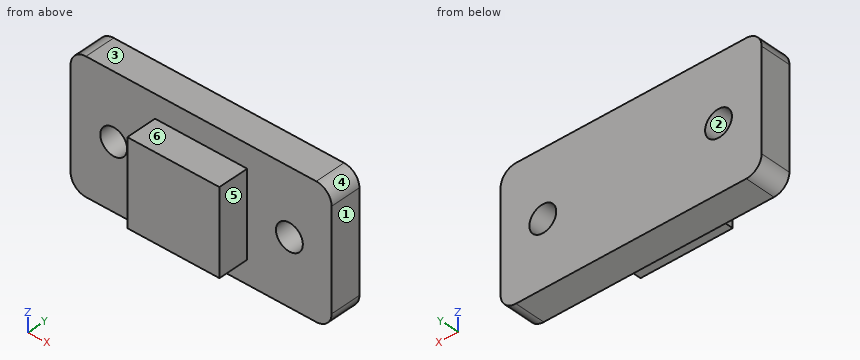
```python
from build123d import *

# Parameters (mm, degrees)
SKETCH1_W           = 12
SKETCH1_H           = 11
BOSS_EXTRUDE1_DEPTH = 4
SKETCH2_W           = 34
SKETCH2_H           = 17
BOSS_EXTRUDE2_DEPTH = 4
SKETCH3_R           = 1.75
CUT_EXTRUDE1_DEPTH  = 5
FILLET1_R           = 2


with BuildPart() as part:
    # Sketch1 → Boss-Extrude1 (new body)
    with BuildSketch(Plane(origin=(0, 0, 0), x_dir=(1, 0, 0), z_dir=(0, 1, 0))):
        with Locations((6, -5.5)):
            Rectangle(SKETCH1_W, SKETCH1_H)
    extrude(amount=BOSS_EXTRUDE1_DEPTH)

    # Sketch2 → Boss-Extrude2 (add)
    with BuildSketch(Plane(origin=(0, 4, 0), x_dir=(1, 0, 0), z_dir=(0, 1, 0))):
        with Locations((6, -5.5)):
            Rectangle(SKETCH2_W, SKETCH2_H)
    extrude(amount=BOSS_EXTRUDE2_DEPTH)

    # Sketch3 → Cut-Extrude1 (cut, through all)
    with BuildSketch(Plane.XZ.offset(-4)):
        with Locations((-5.385399537, 5.5)):
            Circle(SKETCH3_R)
        with Locations((17.5, 5.5)):
            Circle(SKETCH3_R)
    extrude(amount=-CUT_EXTRUDE1_DEPTH, mode=Mode.SUBTRACT)

    # Fillet1
    fillet1_edges = [part.edges().sort_by_distance(p)[0] for p in [
        (23, 6, 14),
        (23, 6, -3),
        (-11, 6, -3),
        (-11, 6, 14),
    ]]
    fillet(fillet1_edges, radius=FILLET1_R)


solid = part.part
```
For this review, take the finished solid that the model builds, in its own axes (mm). Face numbers are marked on the shaded views. A direction names the side the tool comes from. Give positions to 0.01 mm unless a question says otherwise; leave off trailing zeros. Loops run counter-clockwise (first coordinate to the right, second up) from the corner with the lowest first, then second, coordinate; pieces in that order, holes last. Notation, with made-up numbers: M -28,-19.75 L 14,-19.75 A8 cw 14,-7.75 Z; hole C 17.5,-9 d7. An arc over 180 degrees is marked long. One line per item, written item: value. Start each with the question number.
Q1. Machinability: for the marked faces 4, 5 and 6, which of the approach directions +Z, -Z, +X, -X, +Y, -Y give a long, thin tool a straight path to every point of the face, cutting with its end or side? Answer none if there is none.
Q2. Add section C-C (y = 6). Give the boundary of the cut face in (x, z).
Q3. Add section D-D (z = 1.25). Give the boundary of the cut face in (x, y).
Q4. For L1, parallel to Z at x = 17.5, y = 6.5; L2, parallel to X at y = 5.5, z = 4.75; L3, parallel to Z at x = 9.5, y = 0.5, list the stretches that pass through material, from the lowest coordinate up.
Q5. Draft analysis for pull direction Z (two halves, no side actions). For the marked faces 1, 2 and 3, state which applies: released by +Z, released by -Z, zero draft, split by the parting line, or undercut.
Q6. Add section A-A (z = 5.5). Give the boundary of the cut face in (x, y), and give its area (3 significant figures).
Q7. Add section B-B (x = 17.5). Give the boundary of the cut face in (y, z), and give its area (3 significant figures).
Q8. Clearance check with flat-ended pins moving along their axes: pin 1 Ø1.5 at (x, y) = (-6.5, 2.5) entering from +Z; pin 2 Ø1.2 at (x, y) = (9, 1.5) entering from +Z; pin 3 Ø1.2 at (y, z) = (1.5, 7.5) entering from -X; pin 4 Ø1.5 at (y, z) = (2, 6) entering from +X. State where each tip first meets the part, or that it passes through.
Reply:
1. face 4: +Z, +X, +Y, -Y
1. face 5: +Z, -Z, +X, -Y
1. face 6: +Z, +X, -X, -Y
2. outline: M -11,-1 A2 ccw -9,-3 L 21,-3 A2 ccw 23,-1 L 23,12 A2 ccw 21,14 L -9,14 A2 ccw -11,12 Z; hole C -5.39,5.5 d3.5; hole C 17.5,5.5 d3.5
3. outline: M -11,4 L 0,4 L 0,0 L 12,0 L 12,4 L 23,4 L 23,8 L -11,8 Z
4. L1: -3 to 3.75, 7.25 to 14
4. L2: -11 to -6.97, -3.8 to 15.92, 19.08 to 23
4. L3: 0 to 11
5. face 1: zero draft
5. face 2: undercut
5. face 3: released by +Z
6. outline: M -11,4 L -7.14,4 L -7.14,8 L -11,8 Z; M -3.64,4 L 0,4 L 0,0 L 12,0 L 12,4 L 15.75,4 L 15.75,8 L -3.64,8 Z; M 19.25,4 L 23,4 L 23,8 L 19.25,8 Z
6. area: 156 mm²
7. outline: M 4,-3 L 8,-3 L 8,3.75 L 4,3.75 Z; M 4,7.25 L 8,7.25 L 8,14 L 4,14 Z
7. area: 54.0 mm²
8. pin 1: through
8. pin 2: z = 11
8. pin 3: x = 0
8. pin 4: x = 12
